Geometry check sheet. Reference: the model listing, model coordinates, mm. A direction names the side the tool comes from. Coordinates: 2 decimals unless noted, no trailing zeros. Write each loop counter-clockwise with the first axis right and the second up, starting at its lowest first coordinate (ties: lowest second). Pieces come first, ordered by that corner, then holes. Notation, with made-up numbers: (84, 68) -> (138, 68) arc R21 cw to (138, 88) -> close; hole circle Ø9 at (41.5, -24.5). An arc over 180 degrees is marked (long way). Answer in a Markdown table with one row per item. Add a question column.
Q1. Gauge pin test, flat end, axial feed: P1, Ø3, axis at x = 17.5, z = 2.77, coming from the -Y side. Record the tip position at first contact, or that the pin passes through.
Q2. Tool access check on faces 5 (the face through (13, 0, 49)), 6 (the face through (19, 0.99, 1.81)), 7 (the face through (13, 23.4, 49)). Record the directions out of +Z, -Z, +X, -X, +Y, -Y that give a thin tool (end or side, any length) a straight path to the whole face; none if there is none.
Q3. Release check for a two-part mould opening along Z. For faces 1 (the face through (24.4, 13.9, 41.4)), 2 (the face through (24, 13, 0)), 3 (the face through (0, 15, 49)), 4 (the face through (1, 13.9, 41.4)) record: pulls with the +Z half, pulls with the -Z half, needs draft (parallel to the pull), parting line crosses it, or undercut.
Q4. Thickness scan on line 1 (X direction, y = 2.25, z = 55.5); line 2 (Y direction, x = 1.25, z = 45.19) (3 decimals). Record the ranges inside material, lowest first.
Q5. Section check A-A, the plane x = 17.5. Record the boundary of the cut face in (y, z), and give its area (3 significant figures).
Q6. Section check B-B, the plane z = 45.19. Record the boundary of the cut face in (x, y) (3 decimals).
Q7. Section check C-C, the plane x = 22.25. Record the boundary of the cut face in (y, z).
```python
from build123d import *

# Parameters (mm, degrees)
SKETCH1_W           = 25.4
SKETCH1_H           = 25.4
SKETCH1_W_2         = 21.4
SKETCH1_H_2         = 21.4
BOSS_EXTRUDE1_DEPTH = 100
SKETCH2_R           = 3.975
CUT_EXTRUDE1_DEPTH  = 50
SKETCH3_R           = 1.55
CUT_EXTRUDE4_DEPTH  = 10
SKETCH4_R           = 1.778
CUT_EXTRUDE5_DEPTH  = 10
CUT_EXTRUDE6_REACH  = 108.256
SKETCH5_R           = 1.825


with BuildPart() as part:
    # Sketch1 → Boss-Extrude1 (new body)
    with BuildSketch(Plane.XY):
        with Locations((12.7, 12.7)):
            Rectangle(SKETCH1_W, SKETCH1_H)
        with Locations((12.7, 12.7)):
            Rectangle(SKETCH1_W_2, SKETCH1_H_2, mode=Mode.SUBTRACT)
    extrude(amount=BOSS_EXTRUDE1_DEPTH)

    # Sketch2 → Cut-Extrude1 (cut)
    with BuildSketch(Plane(origin=(25.4, 0, 0), x_dir=(0, 0, -1), z_dir=(1, 0, 0))):
        with Locations((-85, 12.7)):
            Circle(SKETCH2_R)
        with Locations((-45.19, 12.7)):
            Circle(SKETCH2_R)
    extrude(amount=-CUT_EXTRUDE1_DEPTH, mode=Mode.SUBTRACT)

    # Sketch3 → Cut-Extrude4 (cut)
    with BuildSketch(Plane.XZ):
        with BuildLine():
            Line((8.45, 10), (8.45, 70))
            ThreePointArc((8.45, 70), (6.9, 68.45), (5.35, 70))
            Line((5.35, 70), (5.35, 10))
            ThreePointArc((5.35, 10), (6.9, 11.55), (8.45, 10))
        make_face()
        with Locations((6.9, 10)):
            Circle(SKETCH3_R)
        with BuildLine():
            ThreePointArc((5.35, 70), (6.9, 68.45), (8.45, 70))
            ThreePointArc((8.45, 70), (6.9, 71.55), (5.35, 70))
        make_face()
    extrude(amount=-CUT_EXTRUDE4_DEPTH, mode=Mode.SUBTRACT)

    # Sketch4 → Cut-Extrude5 (cut)
    with BuildSketch(Plane.XZ):
        with Locations(Location((7.5, 2.765729771, 0), (0, 0, 270))):
            Circle(SKETCH4_R)
        with Locations(Location((17.5, 2.765729771, 0), (0, 0, 270))):
            Circle(SKETCH4_R)
    extrude(amount=-CUT_EXTRUDE5_DEPTH, mode=Mode.SUBTRACT)

    # Cut-Extrude6: up to this face of the body (flat: up to its plane)
    cut_extrude6_end = Plane(part.part.faces().sort_by_distance((25.4, 12.7, 49.385999137))[0])
    # Sketch5 → Cut-Extrude6 (cut, up to the picked face)
    with BuildSketch(Plane.ZY, mode=Mode.PRIVATE) as cut_extrude6_sk1:
        with Locations((7, 12.350192929)):
            Circle(SKETCH5_R)
    cut_extrude6_tool1 = split(extrude(cut_extrude6_sk1.sketch, amount=-CUT_EXTRUDE6_REACH, mode=Mode.PRIVATE), bisect_by=cut_extrude6_end, keep=Keep.BOTH, mode=Mode.PRIVATE)
    add(cut_extrude6_tool1.solids().sort_by(Axis((0, 12.350193, 7), (1, 0, 0)))[0], mode=Mode.SUBTRACT)


solid = part.part
```
Calculated:
| question | item | result |
|---|---|---|
| 1 | P1 | stops at y = 23.4 |
| 2 | face 5 | +Z, -Z, +X, -X, -Y |
| 2 | face 6 | -Y |
| 2 | face 7 | +Z, -Z |
| 3 | face 1 | undercut |
| 3 | face 2 | pulls with the -Z half |
| 3 | face 3 | needs draft |
| 3 | face 4 | undercut |
| 4 | line 1 | x = 0 to 2, 23.4 to 25.4 |
| 4 | line 2 | y = 0 to 8.725, 16.675 to 25.4 |
| 5 | outline | (0, 0) -> (2, 0) -> (2, 0.99) -> (0, 0.99) -> close; (0, 4.54) -> (2, 4.54) -> (2, 100) -> (0, 100) -> close; (23.4, 0) -> (25.4, 0) -> (25.4, 100) -> (23.4, 100) -> close |
| 5 | area | 393 mm² |
| 6 | outline | (0, 0) -> (5.35, 0) -> (5.35, 2) -> (2, 2) -> (2, 8.725) -> (0, 8.725) -> close; (0, 16.675) -> (2, 16.675) -> (2, 23.4) -> (23.4, 23.4) -> (23.4, 16.675) -> (25.4, 16.675) -> (25.4, 25.4) -> (0, 25.4) -> close; (8.45, 0) -> (25.4, 0) -> (25.4, 8.725) -> (23.4, 8.725) -> (23.4, 2) -> (8.45, 2) -> close |
| 7 | outline | (0, 0) -> (2, 0) -> (2, 100) -> (0, 100) -> close; (23.4, 0) -> (25.4, 0) -> (25.4, 100) -> (23.4, 100) -> close |
